Model file for the job. Use its own axes, mm. Face numbers are marked on the shaded views. A direction names the side the tool comes from. Coordinates: 2 decimals unless noted, no trailing zeros. Write each loop counter-clockwise with the first axis right and the second up, starting at its lowest first coordinate (ties: lowest second). Pieces come first, ordered by that corner, then holes. Notation, with made-up numbers: (-25, -9) -> (30, -9) arc R32 cw to (30, 22) -> close; hole circle Ø11 at (-33, 63.25). An arc over 180 degrees is marked (long way). Write item = value, one per line. Start each with the question number.
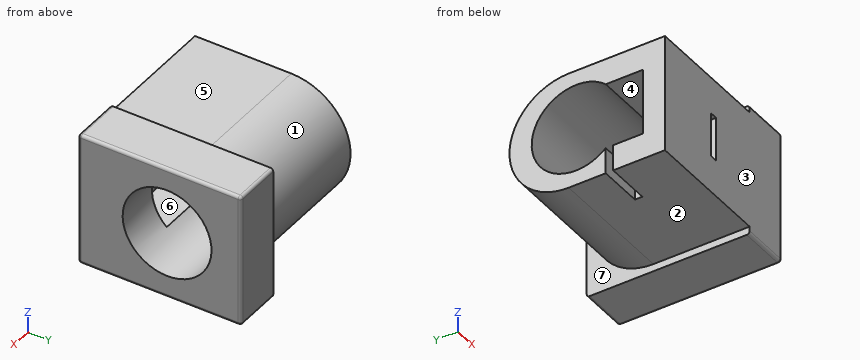
from build123d import *

# Parameters (mm, degrees)
SKETCH1_W               = 9
SKETCH1_H               = 11
BOSS_EXTRUDE1_DEPTH     = 12
CUT_EXTRUDE1_DEPTH      = 1
CUT_EXTRUDE1_DEPTH_BACK = 8.7
SKETCH3_R               = 3
CUT_EXTRUDE2_DEPTH      = 13
CUT_EXTRUDE3_REACH      = 13
SKETCH4_W               = 0.5
SKETCH4_H               = 3
FILLET1_R               = 0.2
CUT_EXTRUDE4_REACH      = 10.5
SKETCH5_W               = 3
SKETCH5_H               = 0.5
SKETCH6_W               = 4.472135954
SKETCH6_H               = 2.5
CUT_EXTRUDE5_DEPTH      = 9


with BuildPart() as part:
    # Sketch1 → Boss-Extrude1 (new body)
    with BuildSketch(Plane(origin=(0, 0, 0), x_dir=(0, 0, -1), z_dir=(1, 0, 0))):
        with Locations((4.5, 5.5)):
            Rectangle(SKETCH1_W, SKETCH1_H)
    extrude(amount=BOSS_EXTRUDE1_DEPTH)

    # Sketch2 → Cut-Extrude1 (cut, two sides)
    with BuildSketch(Plane.ZY) as cut_extrude1_sk:
        with BuildLine():
            Line((-8.5, 0), (-8.5, 6.5))
            ThreePointArc((-8.5, 6.5), (-4.5, 10.5), (-0.5, 6.5))
            Line((-0.5, 6.5), (-0.5, 0))
            Line((-0.5, 0), (0, 0))
            Line((0, 0), (0, 11))
            Line((0, 11), (-9, 11))
            Line((-9, 11), (-9, 0))
            Line((-9, 0), (-8.5, 0))
        make_face()
    extrude(amount=CUT_EXTRUDE1_DEPTH, mode=Mode.SUBTRACT)
    extrude(cut_extrude1_sk.sketch, amount=-CUT_EXTRUDE1_DEPTH_BACK, mode=Mode.SUBTRACT)

    # Sketch3 → Cut-Extrude2 (cut, through all)
    with BuildSketch(Plane(origin=(12, 0, 0), x_dir=(0, 0, -1), z_dir=(1, 0, 0))):
        with Locations((4.5, 6)):
            Circle(SKETCH3_R)
    extrude(amount=-CUT_EXTRUDE2_DEPTH, mode=Mode.SUBTRACT)

    # Sketch4 → Cut-Extrude3 (cut, up to next)
    with BuildSketch(Plane(origin=(0, 0, 0), x_dir=(-1, 0, 0), z_dir=(0, -1, 0)), mode=Mode.PRIVATE) as cut_extrude3_sk1:
        with Locations((-5, 4.5)):
            Rectangle(SKETCH4_W, SKETCH4_H)
    cut_extrude3_tool1 = extrude(cut_extrude3_sk1.sketch, amount=-CUT_EXTRUDE3_REACH, mode=Mode.PRIVATE) & part.part
    add(cut_extrude3_tool1.solids().sort_by_distance((5, 0, -4.5))[0], mode=Mode.SUBTRACT)

    # Fillet1
    fillet1_edges = [part.edges().sort_by_distance(p)[0] for p in [
        (12, 5.5, -9),
        (12, 11, -4.5),
        (12, 5.5, 0),
        (12, 0, -4.5),
        (10.35, 11, 0),
        (10.35, 11, -9),
        (10.35, 0, -9),
        (10.35, 0, 0),
    ]]
    fillet(fillet1_edges, radius=FILLET1_R)

    # Sketch5 → Cut-Extrude4 (cut, up to next)
    with BuildSketch(Plane(origin=(0, 0, -8.5), x_dir=(-1, 0, 0), z_dir=(0, 0, -1)), mode=Mode.PRIVATE) as cut_extrude4_sk1:
        with Locations((-1.5, 3.75)):
            Rectangle(SKETCH5_W, SKETCH5_H)
    cut_extrude4_tool1 = extrude(cut_extrude4_sk1.sketch, amount=-CUT_EXTRUDE4_REACH, mode=Mode.PRIVATE) & part.part
    add(cut_extrude4_tool1.solids().sort_by_distance((1.5, 3.75, -8.5))[0], mode=Mode.SUBTRACT)

    # Sketch6 → Cut-Extrude5 (cut)
    with BuildSketch(Plane.ZY):
        with Locations((-4.5, 2.75)):
            Rectangle(SKETCH6_W, SKETCH6_H)
    extrude(amount=-CUT_EXTRUDE5_DEPTH, mode=Mode.SUBTRACT)


solid = part.part
(1) Saw through at B-B (x = 6.5). Give the cut face in (y, z), then the cut area to 3 significant figures.
(2) Mould opens along Y. For the marked faces 1, 2, 3 and 4 say: released by +Y, released by -Y, zero draft, split by the parting line, or undercut.
(3) Drill centre lines: line 1 along X through (y, z) = (0.5, -4.5); line 2 along Y through (x, z) = (5.75, -4.5); line 3 along Z through (x, y) = (9.5, 6). Where is each one in solid material? Low to high.
(4) Saw through at C-C (z = -4.5). Give the cut face in (x, y), then the cut area to 3 significant figures.
(5) Saw through at D-D (y = 2.5). Give the cut face in (x, z), then the cut area to 3 significant figures.
(6) Saw through at A-A (y = 6). Give the cut face in (x, z).
(7) 3-axis set-ups, long thin cutter, end or side, ignore diameter. For the marked faces 5, 6 and 7: which of +Z, -Z, +X, -X, +Y, -Y reach the whole face in a straight line?
(8) Drop flat-ended pins along their axis: pin 1 Ø5 at (x, z) = (5, -5) entering from +Y; pin 2 Ø1.2 at (x, y) = (5, 2.5) entering from +Z; pin 3 Ø0.5 at (x, z) = (1, -8) entering from +Y. Give the stop position or say it passes through.
Returned:
q1.outline = (0, -8.5) -> (6.5, -8.5) arc R4 ccw to (6.5, -0.5) -> (0, -0.5) -> close; hole (1.5, -6.74) -> (4, -6.74) arc R3 ccw (long way) to (4, -2.26) -> (1.5, -2.26) -> close
q1.area = 40.8 mm2
q2.face_1 = released by +Y
q2.face_2 = zero draft
q2.face_3 = released by -Y
q2.face_4 = undercut
q3.line_1 = 0 to 4.75, 5.25 to 12
q3.line_2 = 0 to 1.5, 9 to 10.5
q3.line_3 = -9 to -7.5, -1.5 to 0
q4.outline = (0, 0) -> (4.75, 0) -> (4.75, 1.5) -> (0, 1.5) -> close; (0, 9) -> (12, 9) -> (12, 10.8) arc R0.2 ccw to (11.8, 11) -> (8.7, 11) -> (8.7, 10.5) -> (0, 10.5) -> close; (5.25, 0) -> (11.8, 0) arc R0.2 ccw to (12, 0.2) -> (12, 3) -> (9, 3) -> (9, 1.5) -> (5.25, 1.5) -> close
q4.area = 41.4 mm2
q5.outline = (0, -8.5) -> (8.7, -8.5) -> (8.7, -9) -> (11.8, -9) arc R0.2 ccw to (12, -8.8) -> (12, -0.2) arc R0.2 ccw to (11.8, 0) -> (8.7, 0) -> (8.7, -0.5) -> (0, -0.5) -> (0, -2.26) -> (9, -2.26) -> (9, -6.74) -> (0, -6.74) -> close
q5.area = 59.0 mm2
q6.outline = (0, -8.5) -> (8.7, -8.5) -> (8.7, -9) -> (11.8, -9) arc R0.2 ccw to (12, -8.8) -> (12, -7.5) -> (0, -7.5) -> close; (0, -1.5) -> (12, -1.5) -> (12, -0.2) arc R0.2 ccw to (11.8, 0) -> (8.7, 0) -> (8.7, -0.5) -> (0, -0.5) -> close
q7.face_5 = +Z, -X, +Y, -Y
q7.face_6 = -X
q7.face_7 = -X, +Y
q8.pin_1 = 10.5
q8.pin_2 = -0.5
q8.pin_3 = 8.83
